```python
from build123d import *

# Parameters (mm, degrees)
SKETCH11_W                     = 3.4
SKETCH11_H                     = 62.2
BASE_FLANGE3_DEPTH             = 30
EDGE_FLANGE1_STRIP_W           = 15.1
EDGE_FLANGE1_STRIP_H           = 3.4
EDGE_FLANGE1_STRIP_CUT_DEPTH   = 30
EDGE_FLANGE1_STRIP_2_W         = 15.1
EDGE_FLANGE1_STRIP_2_H         = 3.4
EDGE_FLANGE1_STRIP_CUT_2_DEPTH = 30
EDGE_FLANGE1_DEPTH             = 30
EDGE_FLANGE1_BEND_DEPTH        = 30
SKETCH22_R                     = 1.5
CUT_EXTRUDE1_DEPTH             = 72.894645141
UNFOLD1_START                  = -20
UNFOLD1_OUTLINE_W              = 62.2
UNFOLD1_OUTLINE_H              = 30
UNFOLD1_DEPTH                  = 16.6
UNFOLD1_START_2                = -3.4
UNFOLD1_2_OUTLINE_W            = 98.637609512
UNFOLD1_2_OUTLINE_H            = 30
UNFOLD1_2_OUTLINE_R            = 1.5
UNFOLD1_2_DEPTH                = 3.4


# Read off the part's stored shape, not the designer's step: Unfold1
# Sheet-metal steps are written as plain solids
with BuildPart() as part:
    # Sketch11 → Base-Flange3 (new body)
    with BuildSketch(Plane.XY):
        with Locations((-1.7, 0)):
            Rectangle(SKETCH11_W, SKETCH11_H)
    extrude(amount=BASE_FLANGE3_DEPTH)

    # Edge-Flange1 strip (across the edge) → Edge-Flange1 strip cut (cut)
    with BuildSketch(Plane(origin=(-3.4, 31.1, 30), x_dir=(0, -1, 0), z_dir=(0, 0, -1))):
        with Locations((-3.4, -1.7)):
            Rectangle(EDGE_FLANGE1_STRIP_W, EDGE_FLANGE1_STRIP_H)
    extrude(amount=EDGE_FLANGE1_STRIP_CUT_DEPTH, mode=Mode.SUBTRACT)

    # Edge-Flange1 strip 2 (across the edge) → Edge-Flange1 strip cut 2 (cut)
    with BuildSketch(Plane(origin=(-3.4, -31.1, 0), x_dir=(0, 1, 0), z_dir=(0, 0, 1))):
        with Locations((-3.4, -1.7)):
            Rectangle(EDGE_FLANGE1_STRIP_2_W, EDGE_FLANGE1_STRIP_2_H)
    extrude(amount=EDGE_FLANGE1_STRIP_CUT_2_DEPTH, mode=Mode.SUBTRACT)

    # Edge-Flange1 section (across the edge) → Edge-Flange1 (add)
    with BuildSketch(Plane(origin=(-3.4, 31.1, 30), x_dir=(0, -1, 0), z_dir=(0, 0, -1))):
        with BuildLine():
            Line((0, 0.75), (0, 16.6))
            Line((0, 16.6), (3.4, 16.6))
            Line((3.4, 16.6), (3.4, 0.75))
            ThreePointArc((3.4, 0.75), (3.619669914, 0.219669914), (4.15, 0))
            Line((4.15, 0), (4.15, -3.4))
            ThreePointArc((4.15, -3.4), (1.215506858, -2.184493142), (0, 0.75))
        make_face()
    extrude(amount=EDGE_FLANGE1_DEPTH)

    # Edge-Flange1 section 2 (across the edge) → Edge-Flange1 bend (add)
    with BuildSketch(Plane(origin=(-3.4, -31.1, 0), x_dir=(0, 1, 0), z_dir=(0, 0, 1))):
        with BuildLine():
            Line((0, 0.75), (0, 16.6))
            Line((0, 16.6), (3.4, 16.6))
            Line((3.4, 16.6), (3.4, 0.75))
            ThreePointArc((3.4, 0.75), (3.619669914, 0.219669914), (4.15, 0))
            Line((4.15, 0), (4.15, -3.4))
            ThreePointArc((4.15, -3.4), (1.215506858, -2.184493142), (0, 0.75))
        make_face()
    extrude(amount=EDGE_FLANGE1_BEND_DEPTH)

    # Sketch22 → Cut-Extrude1 (cut, through all)
    with BuildSketch(Plane(origin=(0, 31.1, 0), x_dir=(1, 0, 0), z_dir=(0, 1, 0))):
        with Locations(Location((-12.329371406, -23.693332437, 0), (0, 0, 180))):
            Circle(SKETCH22_R)
        with Locations(Location((-12.329371406, -6.306667563, 0), (0, 0, 180))):
            Circle(SKETCH22_R)
    extrude(amount=-CUT_EXTRUDE1_DEPTH, mode=Mode.SUBTRACT)

    # Unfold1 outline → Unfold1 (cut)
    with BuildSketch(Plane.YZ.offset(UNFOLD1_START)):
        with Locations((0, 15)):
            Rectangle(UNFOLD1_OUTLINE_W, UNFOLD1_OUTLINE_H)
    extrude(amount=UNFOLD1_DEPTH, mode=Mode.SUBTRACT)

    # Unfold1 2 outline → Unfold1 2 (add)
    with BuildSketch(Plane.YZ.offset(UNFOLD1_START_2)):
        with Locations((0, 15)):
            Rectangle(UNFOLD1_2_OUTLINE_W, UNFOLD1_2_OUTLINE_H)
        with Locations((41.648176162, 23.693332437)):
            Circle(UNFOLD1_2_OUTLINE_R, mode=Mode.SUBTRACT)
        with Locations((41.648176162, 6.306667563)):
            Circle(UNFOLD1_2_OUTLINE_R, mode=Mode.SUBTRACT)
        with Locations((-41.648176162, 23.693332437)):
            Circle(UNFOLD1_2_OUTLINE_R, mode=Mode.SUBTRACT)
        with Locations((-41.648176162, 6.306667563)):
            Circle(UNFOLD1_2_OUTLINE_R, mode=Mode.SUBTRACT)
    extrude(amount=UNFOLD1_2_DEPTH)


solid = part.part
```
For this review, take the finished solid that the model builds, in its own axes (mm). Round coordinates to 2 decimals unless told otherwise and drop trailing zeros. Loops run counter-clockwise (first coordinate to the right, second up) from the corner with the lowest first, then second, coordinate; pieces in that order, holes last.
(1) We need section A-A (y = 41). Give the boundary of the cut face in (x, z).
Returned:
outline: (-3.4, 0) - (0, 0) - (0, 4.95) - (-3.4, 4.95) - close; (-3.4, 7.66) - (0, 7.66) - (0, 22.34) - (-3.4, 22.34) - close; (-3.4, 25.05) - (0, 25.05) - (0, 30) - (-3.4, 30) - close
(2) Clearance check with a flat-ended pin moving along its axis: P1, Ø2.5, axis at y = 41.65, z = 23.69, coming from the -X side. State where the tip first meets the part, or that it passes through.
Returned:
P1: passes through
(3) Wall thickness on line 1 along Z through (x, y) = (-2.55, 42); line 2 along Y through (x, z) = (-1.1, 24): over which ranges is each line inside the solid? List them lowest first.
Returned:
line 1: z = 0 to 4.85, 7.76 to 22.24, 25.15 to 30
line 2: y = -49.32 to -43.12, -40.18 to 40.18, 43.12 to 49.32
(4) Mouldability with a two-part tool opening along Z and no side actions: class faces 1 (the flat face through (-2, -49.319, 15)), 2 (the flat face through (-2, -1, 30)), 3 (the cylindrical face through (-1.724, -40.263, 5.732)) as released by +Z, released by -Z, zero draft, split by the parting line, or undercut.
Returned:
face 1: zero draft
face 2: released by +Z
face 3: undercut
(5) We need section B-B (y = -42). Give the boundary of the cut face in (x, z).
Returned:
outline: (-3.4, 0) - (0, 0) - (0, 4.85) - (-3.4, 4.85) - close; (-3.4, 7.76) - (0, 7.76) - (0, 22.24) - (-3.4, 22.24) - close; (-3.4, 25.15) - (0, 25.15) - (0, 30) - (-3.4, 30) - close
